from build123d import *

# Parameters (mm, degrees)
MODEL_R                  = 8.05
SALIENTE_EXTRUIR1_DEPTH  = 3
CROQUIS2_W               = 3
CROQUIS2_H               = 36.5
SALIENTE_EXTRUIR2_DEPTH  = 15.8
CROQUIS3_R               = 0.75
CROQUIS3_W               = 11.8
CROQUIS3_H               = 22.5
CORTAR_EXTRUIR1_DEPTH    = 3
REDONDEO1_R              = 2
CROQUIS5_R               = 1.5
CORTAR_EXTRUIR3_DEPTH    = 1
REDONDEO1_OF_SIMETR_A1_R = 2
REDONDEO2_R              = 2
CROQUIS6_W               = 20
CROQUIS6_H               = 3
SALIENTE_EXTRUIR3_DEPTH  = 8
CROQUIS7_R               = 1.5
CORTAR_EXTRUIR4_DEPTH    = 3
CROQUIS8_R               = 2.25
CORTAR_EXTRUIR5_DEPTH    = 1
REDONDEO3_R              = 2


with BuildPart() as part:
    # Model → Saliente-Extruir1 (new body)
    with BuildSketch(Plane.XY):
        with BuildLine():
            Line((117.128163256, -122.351547449), (137.128163256, -122.351547449))
            Line((137.128163256, -122.351547449), (137.128163256, -121.037289507))
            ThreePointArc((137.128163256, -121.037289507), (137.713949693, -119.623075945), (139.128163256, -119.037289507))
            Line((139.128163256, -119.037289507), (157.128163256, -119.037289507))
            ThreePointArc((157.128163256, -119.037289507), (158.542376818, -118.45150307), (159.128163256, -117.037289507))
            Line((159.128163256, -117.037289507), (159.128163256, -105.429203673))
            ThreePointArc((159.128163256, -105.429203673), (159.713949693, -104.014990111), (161.128163256, -103.429203673))
            Line((161.128163256, -103.429203673), (168.128163256, -103.429203673))
            Line((168.128163256, -103.429203673), (168.128163256, -66.929203673))
            Line((168.128163256, -66.929203673), (161.128163256, -66.929203673))
            ThreePointArc((161.128163256, -66.929203673), (159.713949693, -66.343417236), (159.128163256, -64.929203673))
            Line((159.128163256, -64.929203673), (159.128163256, -45.925126076))
            ThreePointArc((159.128163256, -45.925126076), (158.525375774, -44.832630562), (157.530270287, -44.079859504))
            ThreePointArc((157.530270287, -44.079859504), (150.626254462, -40.441158757), (148.250928406, -33.007222803))
            ThreePointArc((148.250928406, -33.007222803), (139.057304014, -34.79177863), (130.970368491, -39.515002403))
            ThreePointArc((130.970368491, -39.515002403), (127.01096078, -36.241427472), (124.933546078, -31.542752084))
            ThreePointArc((124.933546078, -31.542752084), (119.585499261, -33.477559346), (115.007991873, -36.852690455))
            ThreePointArc((115.007991873, -36.852690455), (113.960942039, -34.357491642), (114.984938003, -31.852743603))
            ThreePointArc((114.984938003, -31.852743603), (108.346137898, -34.269313364), (103.017340976, -38.907998482))
            ThreePointArc((103.017340976, -38.907998482), (102.522640368, -36.230932008), (103.164365263, -33.585255769))
            ThreePointArc((103.164365263, -33.585255769), (97.657864433, -36.973852922), (95.128163256, -42.924042331))
            Line((95.128163256, -42.924042331), (95.128163256, -64.929203673))
            ThreePointArc((95.128163256, -64.929203673), (94.542376818, -66.343417236), (93.128163256, -66.929203673))
            Line((93.128163256, -66.929203673), (86.128163256, -66.929203673))
            Line((86.128163256, -66.929203673), (86.128163256, -103.429203673))
            Line((86.128163256, -103.429203673), (93.128163256, -103.429203673))
            ThreePointArc((93.128163256, -103.429203673), (94.542376818, -104.014990111), (95.128163256, -105.429203673))
            Line((95.128163256, -105.429203673), (95.128163256, -117.046472124))
            ThreePointArc((95.128163256, -117.046472124), (95.687839985, -118.507520387), (97.128163256, -119.118559619))
            Line((97.128163256, -119.118559619), (115.128163256, -119.118559619))
            ThreePointArc((115.128163256, -119.118559619), (116.542376818, -119.704346056), (117.128163256, -121.118559619))
            Line((117.128163256, -121.118559619), (117.128163256, -122.351547449))
        make_face()
        with Locations((114.128163256, -55.929203673)):
            Circle(MODEL_R, mode=Mode.SUBTRACT)
        with Locations((140.128163256, -55.929203673)):
            Circle(MODEL_R, mode=Mode.SUBTRACT)
        Polygon((143.127299166, -104.206170984), (143.127299166, -71.873604522), (111.129027345, -71.873604522), (111.129027345, -103.873604522), align=None, mode=Mode.SUBTRACT)
    extrude(amount=SALIENTE_EXTRUIR1_DEPTH)

    # Croquis2 → Saliente-Extruir2 (add)
    with BuildSketch(Plane(origin=(0, 0, 0), x_dir=(-1, 0, 0), z_dir=(0, 0, -1))):
        with Locations((-166.628163256, -85.179203673)):
            Rectangle(CROQUIS2_W, CROQUIS2_H)
    saliente_extruir2 = extrude(amount=SALIENTE_EXTRUIR2_DEPTH)

    # Croquis3 → Cortar-Extruir1 (cut)
    with BuildSketch(Plane(origin=(168.128163256, 0, 0), x_dir=(0, 0, -1), z_dir=(1, 0, 0))):
        with Locations((7.9, -98.829203673)):
            Circle(CROQUIS3_R)
        with Locations((7.9, -71.529203673)):
            Circle(CROQUIS3_R)
        with Locations((7.9, -85.179203673)):
            Rectangle(CROQUIS3_W, CROQUIS3_H)
    cortar_extruir1 = extrude(amount=-CORTAR_EXTRUIR1_DEPTH, mode=Mode.SUBTRACT)

    # Redondeo1
    redondeo1_edges = [part.edges().sort_by_distance(p)[0] for p in [
        (166.628163256, -103.429203673, -15.8),
        (166.628163256, -66.929203673, -15.8),
    ]]
    fillet(redondeo1_edges, radius=REDONDEO1_R)

    # Croquis5 → Cortar-Extruir3 (cut)
    with BuildSketch(Plane(origin=(168.128163256, 0, 0), x_dir=(0, 0, -1), z_dir=(1, 0, 0))):
        with Locations((7.9, -71.529203673)):
            Circle(CROQUIS5_R)
        with Locations((7.9, -98.829203673)):
            Circle(CROQUIS5_R)
    cortar_extruir3 = extrude(amount=-CORTAR_EXTRUIR3_DEPTH, mode=Mode.SUBTRACT)

    # Simetría1: Saliente-Extruir2, Cortar-Extruir1, Cortar-Extruir3 across plane
    add(saliente_extruir2.mirror(Plane(origin=(127.128163256, 0, 0), x_dir=(0, 0, 1), z_dir=(1, 0, 0))))
    add(cortar_extruir1.mirror(Plane(origin=(127.128163256, 0, 0), x_dir=(0, 0, 1), z_dir=(1, 0, 0))), mode=Mode.SUBTRACT)
    add(cortar_extruir3.mirror(Plane(origin=(127.128163256, 0, 0), x_dir=(0, 0, 1), z_dir=(1, 0, 0))), mode=Mode.SUBTRACT)

    # Redondeo1 of Simetría1
    redondeo1_of_simetr_a1_edges = [part.edges().sort_by_distance(p)[0] for p in [
        (87.628163256, -103.429203673, -15.8),
        (87.628163256, -66.929203673, -15.8),
    ]]
    fillet(redondeo1_of_simetr_a1_edges, radius=REDONDEO1_OF_SIMETR_A1_R)

    # Redondeo2
    redondeo2_edges = [part.edges().sort_by_distance(p)[0] for p in [
        (168.128163256, -85.179203673, 3),
        (86.128163256, -85.179203673, 3),
    ]]
    fillet(redondeo2_edges, radius=REDONDEO2_R)

    # Croquis6 → Saliente-Extruir3 (add)
    with BuildSketch(Plane(origin=(0, 0, 0), x_dir=(-1, 0, 0), z_dir=(0, 0, -1))):
        with Locations((-127.128163256, -120.851547449)):
            Rectangle(CROQUIS6_W, CROQUIS6_H)
    extrude(amount=SALIENTE_EXTRUIR3_DEPTH)

    # Croquis7 → Cortar-Extruir4 (cut)
    with BuildSketch(Plane(origin=(0, -119.351547449, 0), x_dir=(1, 0, 0), z_dir=(0, 1, 0))):
        with Locations((133.128163256, 3.5)):
            Circle(CROQUIS7_R)
        with Locations((121.128163256, 3.5)):
            Circle(CROQUIS7_R)
    extrude(amount=-CORTAR_EXTRUIR4_DEPTH, mode=Mode.SUBTRACT)

    # Croquis8 → Cortar-Extruir5 (cut)
    with BuildSketch(Plane(origin=(0, -119.351547449, 0), x_dir=(1, 0, 0), z_dir=(0, 1, 0))):
        with Locations((133.128163256, 3.5)):
            Circle(CROQUIS8_R)
        with Locations((121.128163256, 3.5)):
            Circle(CROQUIS8_R)
    extrude(amount=-CORTAR_EXTRUIR5_DEPTH, mode=Mode.SUBTRACT)

    # Redondeo3
    redondeo3_edges = [part.edges().sort_by_distance(p)[0] for p in [
        (117.128163256, -120.851547449, -8),
        (137.128163256, -120.851547449, -8),
    ]]
    fillet(redondeo3_edges, radius=REDONDEO3_R)


solid = part.part
Could you check a few things on this model? Use its own coordinates, in mm. A direction names the side the tool comes from. Give positions to 0.01 mm unless a question says otherwise; leave off trailing zeros. Order: outer loops, then holes, each group sorted by start corner. A loop starts at its lowest first (then second) coordinate and runs counter-clockwise, first axis right, second up. Notation, with made-up numbers: (4.25, -33.5) - (34.25, -33.5) arc R20 ccw to (34.25, -26.5) - close; hole circle Ø9 at (-23.5, -4). An arc over 180 degrees is marked (long way). Return JSON: item names as keys, results as strings. Group by question number.
Q1. Suppose I cut it at A-A, the plane y = -84. Please give me the cut outline in (x, z).
Q2. Will these pins go through, and if not, where does the flat tip stop? pin 1 Ø2.5 at (y, z) = (-98.83, -7.9) entering from -X; pin 2 Ø2 at (x, z) = (132.5, -2.5) entering from +Y; pin 3 Ø3 at (x, z) = (150.5, 1) entering from +Y; pin 4 Ø12 at (x, y) = (125, -92.5) entering from -Z.
Q3. Thinking about a two-plate mould opening in X: for faces 6 (the face through (130.88, -119.84, -3.6)), 7 (the face through (117.128, -121, -2)), 8 (the face through (88, -85, -13.8)), which applies, pulls with the +X half, pulls with the -X half, needs draft (parallel to the pull), parting line crosses it, or undercut?
Q4. Which directions (+Z, -Z, +X, -X, +Y, -Y) give clear straight access to the entire face, cutting with the end or side of a thin tool? Please do faces 1 (the face through (143.127, -88, 1)), 2 (the face through (122, -120.352, -2)), 3 (the face through (88, -96.429, -8)), 4 (the face through (165.128, -85, -15)), 5 (the face through (167.128, -99, -7)).
Q5. Suppose I cut it at B-B, the plane x = 129. Please give me the cut outline in (y, z).
Q6. Suppose I cut it at C-C, the plane z = -3.5. State how many separate pieces and enclosed holes the cut face has, and give its area (3 significant figures).
Q7. Please list where these lines run through material, in increasing order: line 1 along X through (y, z) = (-121.1, -3.5); line 2 along X through (y, z) = (-72.5, -9.25); line 3 along Y through (x, z) = (135, 1.75). Write a range as [from, to].
Q8. Suppose I cut it at D-D, the plane y = -116. Please give me the cut outline in (x, z), and give its area (3 significant figures).
Resolved:
{
 "1": {"outline": "(86.13, -15.8) - (89.13, -15.8) - (89.13, -13.8) - (86.13, -13.8) - close; (86.13, -2) - (89.13, -2) - (89.13, 0) - (111.13, 0) - (111.13, 3) - (88.13, 3) arc R2 ccw to (86.13, 1) - close; (143.13, 0) - (165.13, 0) - (165.13, -2) - (168.13, -2) - (168.13, 1) arc R2 ccw to (166.13, 3) - (143.13, 3) - close; (165.13, -15.8) - (168.13, -15.8) - (168.13, -13.8) - (165.13, -13.8) - close"},
 "2": {"pin 1": "stops at x = 87.13", "pin 2": "stops at y = -120.35", "pin 3": "stops at y = -37.76", "pin 4": "passes through"},
 "3": {"face 6": "undercut", "face 7": "pulls with the -X half", "face 8": "needs draft"},
 "4": {"face 1": "+Z, -Z", "face 2": "+Y", "face 3": "+X, -X", "face 4": "-Z, +Y, -Y", "face 5": "+X"},
 "5": {"outline": "(-122.35, -8) - (-119.35, -8) - (-119.35, 0) - (-104.06, 0) - (-104.06, 3) - (-122.35, 3) - close; (-71.87, 0) - (-38.27, 0) - (-38.27, 3) - (-71.87, 3) - close"},
 "6": {"separate pieces": "7", "enclosed holes": "0", "area": "123 mm2"},
 "7": {"line 1": "x = [117.13, 119.63], [122.63, 131.63], [134.63, 137.13]", "line 2": "x = [86.13, 89.13], [165.13, 168.13]", "line 3": "y = [-122.35, -104.12], [-71.87, -62.13], [-49.72, -36.7]"},
 "8": {"outline": "(95.13, 0) - (159.13, 0) - (159.13, 3) - (95.13, 3) - close", "area": "192 mm2"}
}
